For this review, use the dimensioned drawing (mm, ordinates from the lowest corner) and the shaded views. Give positions to 0.01 mm unless a question says otherwise; leave off trailing zeros. Write each loop counter-clockwise with the first axis right and the second up, starting at its lowest first coordinate (ties: lowest second). Pieces come first, ordered by that corner, then holes. Notation, with made-up numbers: (21.5, -24.5) -> (47.5, -24.5) arc R7 cw to (47.5, -15.5) -> close; hole circle Ø3 at (-18.75, 2). An arc over 180 degrees is marked (long way). Return JSON: item names as keys, results as strings.
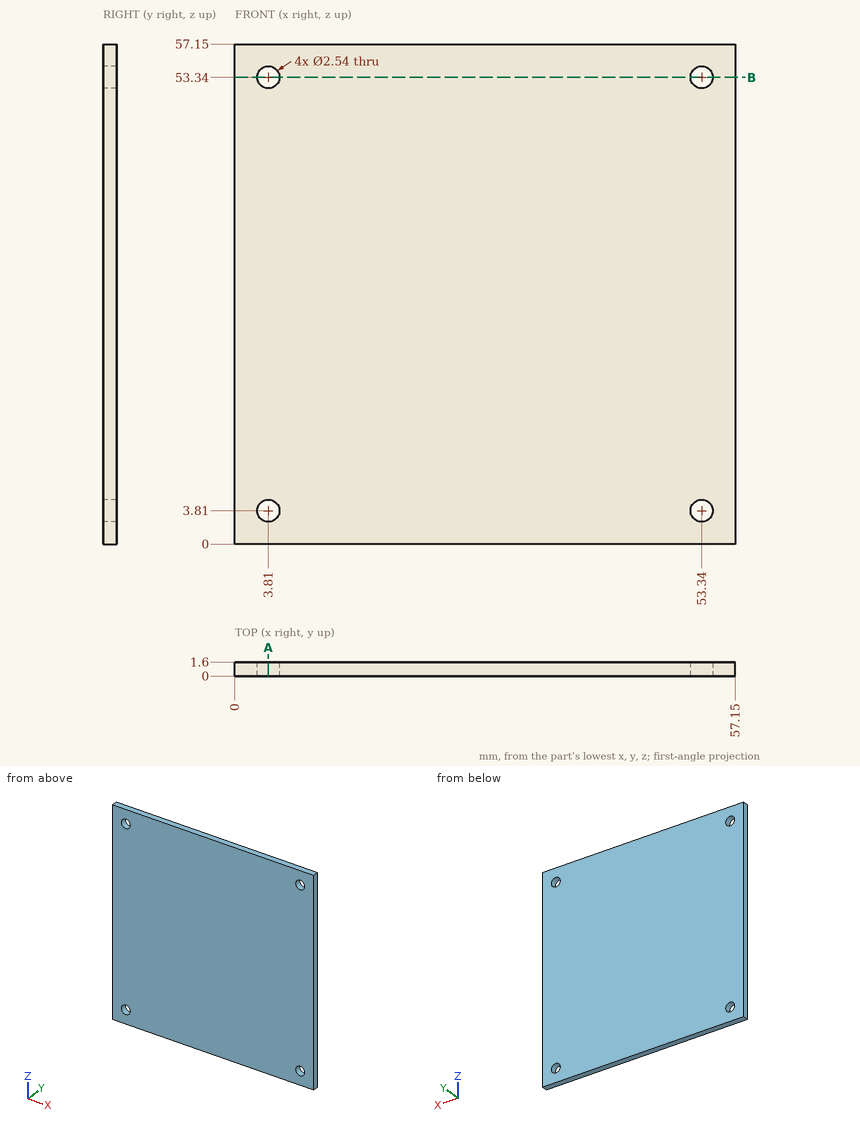
1. Add section B-B, the plane z = 53.34. State the section outline as (x, y) points.
Results found:
{"outline": "(0, 0) -> (2.54, 0) -> (2.54, 1.6) -> (0, 1.6) -> close; (5.08, 0) -> (52.07, 0) -> (52.07, 1.6) -> (5.08, 1.6) -> close; (54.61, 0) -> (57.15, 0) -> (57.15, 1.6) -> (54.61, 1.6) -> close"}
2. Add section A-A, the plane x = 3.81. State the section outline as (y, z) points, plus the area to 3 significant figures.
Results found:
{"outline": "(0, 0) -> (1.6, 0) -> (1.6, 2.54) -> (0, 2.54) -> close; (0, 5.08) -> (1.6, 5.08) -> (1.6, 52.07) -> (0, 52.07) -> close; (0, 54.61) -> (1.6, 54.61) -> (1.6, 57.15) -> (0, 57.15) -> close", "area": "83.3 mm²"}
3. To check wall thickness, follow probe 1 along X at (y, z) = (0.85, 53.34); probe 2 along X at (y, z) = (0.6, 4). State the ranges of each line that lie inside material, in increasing order.
Results found:
{"probe 1": "x = 0 to 2.54, 5.08 to 52.07, 54.61 to 57.15", "probe 2": "x = 0 to 2.55, 5.07 to 52.08, 54.6 to 57.15"}
